Input: dimensioned drawing with shaded views. Units: mm. Origin: part minimum x, y, z. Round coordinates to 2 decimals unless told otherwise and drop trailing zeros. Loops run counter-clockwise (first coordinate to the right, second up) from the corner with the lowest first, then second, coordinate; pieces in that order, holes last. Notation, with made-up numbers: (42.25, 17.25) - (61.25, 17.25) arc R11 cw to (61.25, 38.25) - close; hole circle Ø6 at (17, 82). An arc over 180 degrees is marked (long way). One line per question, with ' | ' between items. Start each with the question number.
1. Cut plane C-C (z = 3.9). Return loops of the section in (x, y), then the cut area to 3 significant figures.
2. Cut plane B-B (y = 4.35). Return loops of the section in (x, z), then the cut area to 3 significant figures.
3. Pin query (flat end, axial travel): pin 1 (5 mm diameter, centred on x = 15, y = 4.35, fed in from -Z). Return the tip coordinate at first contact, or that it passes through.
4. Mould query, pull axis X, two halves, no side actions, for the marked faces 1, 2, 3 and 4. Classes: pulls with the +X half, pulls with the -X half, needs draft (parallel to the pull), parting line crosses it, or undercut.
5. Cut plane A-A (x = 15). Return loops of the section in (y, z), then the cut area to 3 significant figures.
6. Ray query, line 1 (Y direction, x = 15, z = 1.65); line 2 (X direction, y = 4.25, z = 1.65); line 3 (Y direction, x = 14, z = 4.3). Return the intervals inside material, ascending.
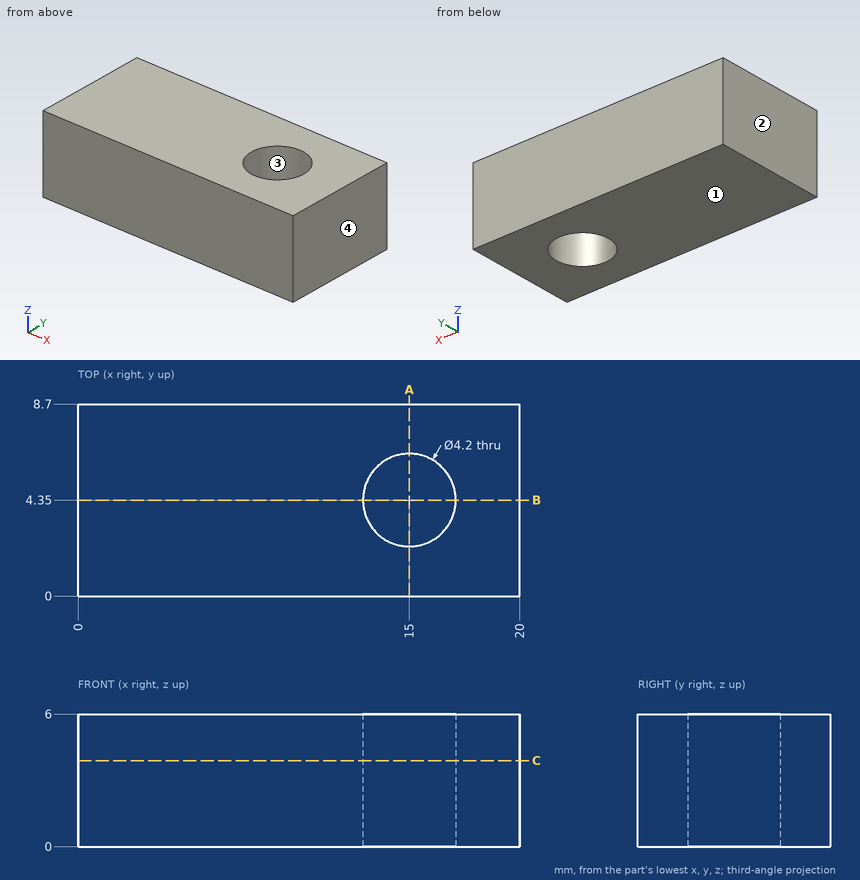
Answers follow:
1) outline: (0, 0) - (20, 0) - (20, 8.7) - (0, 8.7) - close; hole circle Ø4.2 at (15, 4.35) | area: 160 mm2
2) outline: (0, 0) - (12.9, 0) - (12.9, 6) - (0, 6) - close; (17.1, 0) - (20, 0) - (20, 6) - (17.1, 6) - close | area: 94.8 mm2
3) pin 1: stops at z = 0
4) face 1: needs draft | face 2: pulls with the -X half | face 3: undercut | face 4: pulls with the +X half
5) outline: (0, 0) - (2.25, 0) - (2.25, 6) - (0, 6) - close; (6.45, 0) - (8.7, 0) - (8.7, 6) - (6.45, 6) - close | area: 27.0 mm2
6) line 1: y = 0 to 2.25, 6.45 to 8.7 | line 2: x = 0 to 12.9, 17.1 to 20 | line 3: y = 0 to 2.5, 6.2 to 8.7
